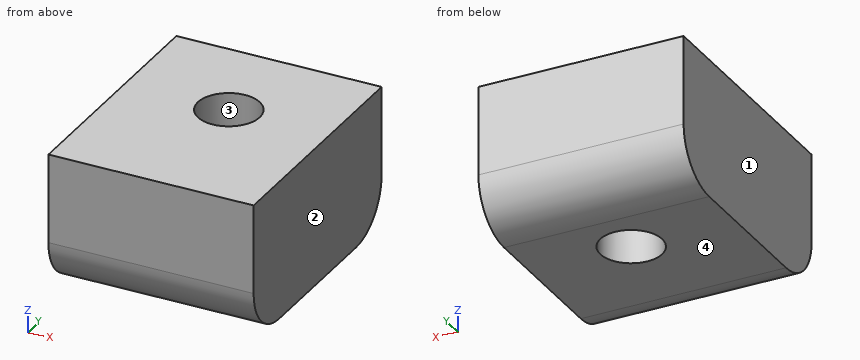
```python
from build123d import *

# Parameters (mm, degrees)
F0_W     = 21.076461
F0_H     = 14.229262
F1_DEPTH = 25.4
F2_R     = 5.08
F4_D     = 6.35
F5_R     = 5.08


with BuildPart() as f1:
    # F0 (on Front) → F1 (new body)
    with BuildSketch(Plane.XZ):
        with Locations((10.53823, 7.114631)):
            Rectangle(F0_W, F0_H)
    extrude(amount=F1_DEPTH)

    # F2
    f2_edges = [f1.edges().sort_by_distance(p)[0] for p in [
        (10.538231, -25.4, 0),
    ]]
    fillet(f2_edges, radius=F2_R)

    # F4 (through all)
    with Locations(Plane(origin=(0, 0, 0), x_dir=(1, 0, 0), z_dir=(0, 0, -1))):
        with Locations((10.692811, 10.257974)):
            Hole(F4_D / 2)

    # F5
    f5_edges = [f1.edges().sort_by_distance(p)[0] for p in [
        (10.538231, 0, 0),
    ]]
    fillet(f5_edges, radius=F5_R)


solid = f1.part
```
Geometry check sheet. Reference: the model listing, model coordinates, mm. Face numbers are marked on the shaded views. Give positions to 0.01 mm unless a question says otherwise; leave off trailing zeros. Loops run counter-clockwise (first coordinate to the right, second up) from the corner with the lowest first, then second, coordinate; pieces in that order, holes last. Notation, with made-up numbers: (-34.75, 47.5) - (-20.75, 47.5) arc R38 cw to (-20.75, 86.5) - close; hole circle Ø10 at (74, 35.25). An arc over 180 degrees is marked (long way). Use CSV: the item, a comma, the result in double quotes. Start each with the question number.
Q1. Release check for a two-part mould opening along X. For the marked faces 1, 2, 3 and 4 record: +X half, -X half, draft (parallel to the pull), parting line (faces both ways), or undercut.
Q2. Section check C-C, the plane z = 6. Record the cut outline in (x, y) (3 decimals).
Q3. Go/stop test with a flat-tipped pin: pin 1 Ø8 at (x, z) = (14, 3.5) entering from +Y. Record where the tip stops, or that it passes through.
Q4. Section check B-B, the plane x = 6.75. Record the cut outline in (y, z), and give its area (3 significant figures).
Q5. Section check A-A, the plane y = -11.25. Record the cut outline in (x, z), and give its area (3 significant figures).
Q6. Scan lines: probe 1 along Y at (x, z) = (11.25, 11.5); probe 2 along Y at (x, z) = (11.75, 13); probe 3 along X at (y, z) = (-12, 1). Record each from-to range of solid material in increasing order. Write a range as from..to.
Q7. Section check D-D, the plane y = -2. Record the cut outline in (x, z).
Findings below:
1,face 1,"-X half"
1,face 2,"+X half"
1,face 3,"undercut"
1,face 4,"draft"
2,outline,"(0, -25.4) - (21.076, -25.4) - (21.076, 0) - (0, 0) - close; hole circle Ø6.35 at (10.693, -10.258)"
3,pin 1,"stops at y = 0"
4,outline,"(-25.4, 5.08) arc R5.08 ccw to (-20.32, 0) - (-5.08, 0) arc R5.08 ccw to (0, 5.08) - (0, 14.23) - (-25.4, 14.23) - close"
4,area,"350 mm^2"
5,outline,"(0, 0) - (7.68, 0) - (7.68, 14.23) - (0, 14.23) - close; (13.71, 0) - (21.08, 0) - (21.08, 14.23) - (13.71, 14.23) - close"
5,area,"214 mm^2"
6,probe 1,"y = -25.4..-13.38, -7.13..0"
6,probe 2,"y = -25.4..-13.25, -7.26..0"
6,probe 3,"x = 0..8.04, 13.35..21.08"
7,outline,"(0, 1.04) - (21.08, 1.04) - (21.08, 14.23) - (0, 14.23) - close"
